Geometry: see drawing. Coordinates: mm, zero at the bounding-box minimum. A direction names the side the tool comes from. Give positions to 0.01 mm unless a question says otherwise; leave off trailing zeros. Order: outer loops, then holes, each group sorted by start corner. A loop starts at its lowest first (then second) coordinate and runs counter-clockwise, first axis right, second up. Notation, with made-up numbers: M 22.5,9 L 78.5,9 A10 ccw 78.5,22 Z; hole C -19,61 d11. An arc over 180 degrees is marked long. Answer as a JSON object with one key per item and string values. Group by question number.
1. Section query A-A (z = 14). Output: boundary loops of the cut face in (x, y) (3 decimals), plus the area to 3 significant figures.
2. Section query B-B (x = 14). Output: boundary loops of the cut face in (y, z) (3 decimals), plus the area to 3 significant figures.
3. Section query C-C (y = 19). Output: boundary loops of the cut face in (x, z).
4. Pin query (flat end, axial travel): P1, Ø1.8, axis at y = 12.5, z = 13, coming from the +X side; P2, Ø1.8, axis at x = 3.5, z = 14, coming from the +Y side; P3, Ø5.5, axis at x = 14, y = 14, coming from the +Z side. Return the tip coordinate at first contact, or that it passes through.
5. Set-up query: the marked faces 5, 6 and 7. Return all of +Z, -Z, +X, -X, +Y, -Y with unobstructed straight access to the full face (end or side cutting, diameter ignored); none if empty.
6. Pull-direction query (Y, two-part tool) for the marked faces 1, 2, 3 and 4; classes: +Y half, -Y half, draft (parallel to the pull), parting line (faces both ways), or undercut.
7. Section query D-D (x = 19.75). Output: boundary loops of the cut face in (y, z), plus the area to 3 significant figures.
8. Material intervals for L1, parallel to Y at x = 14, z = 21.75; L2, parallel to Y at x = 14, z = 4.5 (3 decimals); L3, parallel to Z at x = 7.75, y = 11.5, sorted ascending. Write a range as [from, to].
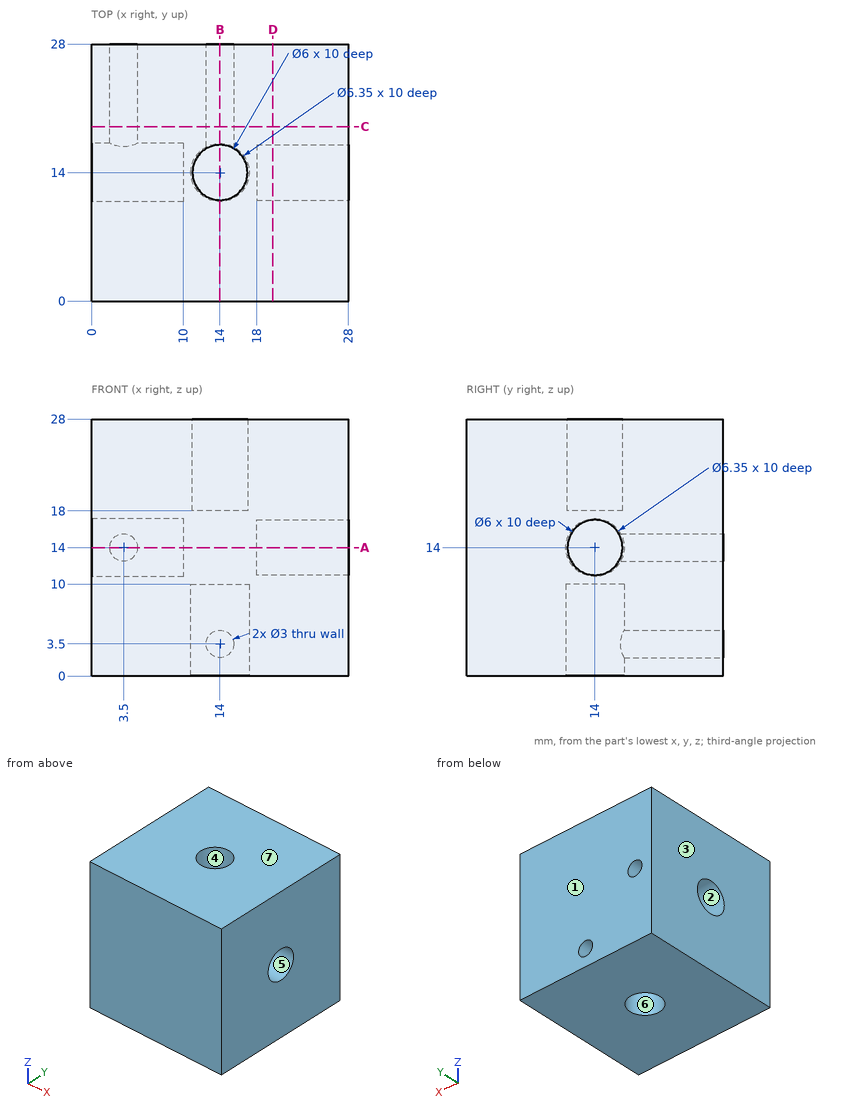
Answer sheet:
{
 "1": {"outline": "M 0,0 L 28,0 L 28,11 L 18,11 L 18,17 L 28,17 L 28,28 L 5,28 L 5,17.175 L 10,17.175 L 10,10.825 L 0,10.825 Z; M 0,17.175 L 2,17.175 L 2,28 L 0,28 Z", "area": "628 mm^2"},
 "2": {"outline": "M 0,0 L 10.825,0 L 10.825,10 L 17.175,10 L 17.175,5 L 28,5 L 28,28 L 17,28 L 17,18 L 11,18 L 11,28 L 0,28 Z; M 17.175,0 L 28,0 L 28,2 L 17.175,2 Z", "area": "628 mm^2"},
 "3": {"outline": "M 0,0 L 28,0 L 28,28 L 0,28 Z; hole C 3.5,14 d3; hole C 14,3.5 d3"},
 "4": {"P1": "x = 18", "P2": "y = 10.96", "P3": "z = 18"},
 "5": {"face 5": "+X", "face 6": "-Z", "face 7": "+Z, +X, -X, +Y, -Y"},
 "6": {"face 1": "+Y half", "face 2": "undercut", "face 3": "draft", "face 4": "undercut"},
 "7": {"outline": "M 0,0 L 28,0 L 28,28 L 0,28 Z; hole C 14,14 d6", "area": "756 mm^2"},
 "8": {"L1": "[0, 11], [17, 28]", "L2": "[0, 10.825]", "L3": "[0, 12.04], [15.96, 28]"}
}
